For this review, take the finished solid that the model builds, in its own axes (mm). A direction names the side the tool comes from. Round coordinates to 2 decimals unless told otherwise and drop trailing zeros. Order: outer loops, then holes, each group sorted by start corner. A loop starts at its lowest first (then second) coordinate and runs counter-clockwise, first axis right, second up. Notation, with made-up numbers: (53.5, -3.5) - (65.5, -3.5) arc R21 cw to (65.5, 28.5) - close; hole circle Ø8 at (73, 4.5). An arc over 180 degrees is marked (long way). One line per item, written item: value.
Autodesk Inventor part; units mm, degrees
ref_plane "YZ Plane" through (0, 0, 0) normal (1, 0, 0) x (0, 1, 0)
ref_plane "XZ Plane" through (0, 0, 0) normal (0, 1, 0) x (-1, 0, 0)
ref_plane "XY Plane" through (0, 0, 0) normal (0, 0, 1) x (1, 0, 0)
sketch "Sketch1" plane through (0, 0, 0) normal (0, 1, 0) x (-1, 0, 0)
  line L0 (53.975, 34.925) -> (-53.975, 34.925)
  line L1 (-53.975, 34.925) -> (-53.975, -34.925)
  line L2 (-53.975, -34.925) -> (53.975, -34.925)
  line L3 (53.975, -34.925) -> (53.975, 34.925)
  line L4 (0, -48.895) -> (0, 48.895)
  line L5 (-75.565, 0) -> (75.565, 0)
  point P0 (0, 0)
  dimension "d0" = 69.85
  dimension "d1" = 107.95
extrude "Extrusion1" add sketch "Sketch1" along normal blind 50.8
sketch "Sketch2" plane through (0, 50.8, 0) normal (0, 1, 0) x (1, 0, 0)
  line L0 (-53.975, -34.925) -> (53.975, -34.925)
  line L1 (53.975, -34.925) -> (53.975, 34.925)
  line L2 (53.975, 34.925) -> (-53.975, 34.925)
  line L3 (-53.975, 34.925) -> (-53.975, -34.925)
  line L4 (15.875, -9.525) -> (41.275, -9.525)
  line L5 (41.275, -9.525) -> (41.275, 9.525)
  line L6 (41.275, 9.525) -> (15.875, 9.525)
  line L7 (15.875, 9.525) -> (15.875, -9.525)
  line L8 (75.565, 0) -> (-75.565, 0)
  circle A0 centre (28.575, 0) radius 3.175
  line L9 (28.575, -9.525) -> (28.575, 9.525) construction
  point P0 (0, 0)
  dimension "d4" = 25.4
  dimension "d5" = 19.05
  dimension "d7" = 6.35
  dimension "d29" = 12.7
extrude "Extrusion2" add sketch "Sketch2" along normal blind 28.575 contours L8 A0 L5 L4 L7 | L7 L6 L5 L8 A0
sketch "Sketch3" plane through (-53.975, 0, -34.925) normal (-1, 0, 0) x (0, 0, 1)
  line L0 (0, 0) -> (69.85, 0)
  line L1 (69.85, 0) -> (69.85, 50.8)
  line L2 (0, 50.8) -> (69.85, 50.8)
  line L3 (0, 0) -> (0, 50.8)
  line L4 (65.278, 4.572) -> (4.572, 4.572)
  line L5 (4.572, 4.572) -> (4.572, 46.228)
  line L6 (4.572, 46.228) -> (65.278, 46.228)
  line L7 (65.278, 46.228) -> (65.278, 4.572)
  point P0 (34.925, 0)
  dimension "d10" = 4.572
extrude "Extrusion3" cut sketch "Sketch3" against normal up to next contours L4 L5 L6 L7
sketch "Sketch4" plane through (0, 0, 0) normal (0, -1, 0) x (1, 0, 0)
  line L0 (-53.975, 34.925) -> (53.975, 34.925)
  line L1 (-53.975, -34.925) -> (-53.975, 34.925)
  line L2 (53.975, -34.925) -> (-53.975, -34.925)
  line L3 (53.975, 34.925) -> (53.975, -34.925)
  line L4 (9.525, -19.05) -> (47.625, -19.05)
  line L5 (47.625, -19.05) -> (47.625, 19.05)
  line L6 (47.625, 19.05) -> (9.525, 19.05)
  line L7 (9.525, 19.05) -> (9.525, -19.05)
  line L8 (-79.233, 0) -> (97.5728, 0) construction
  arc A0 (-41.275, 9.525) -> (-41.275, -9.525) centre (-41.275, 0) ccw
  arc A1 (-15.875, -9.525) -> (-15.875, 9.525) centre (-15.875, 0) ccw
  arc A2 (-41.275, -23.3807) -> (-41.275, -27.4193) centre (-41.275, -25.4) ccw
  arc A3 (-15.875, -27.4193) -> (-15.875, -23.3807) centre (-15.875, -25.4) ccw
  arc A4 (-41.275, 27.4193) -> (-41.275, 23.3807) centre (-41.275, 25.4) ccw
  arc A5 (-15.875, 23.3807) -> (-15.875, 27.4193) centre (-15.875, 25.4) ccw
  line L9 (-28.575, -34.925) -> (-28.575, 34.925) construction
  line L10 (-41.275, -25.4) -> (-41.275, 25.4) construction
  line L11 (-41.275, -27.4193) -> (-15.875, -27.4193)
  line L12 (-15.875, -23.3807) -> (-41.275, -23.3807)
  line L13 (-41.275, 23.3807) -> (-15.875, 23.3807)
  line L14 (-15.875, 27.4193) -> (-41.275, 27.4193)
  line L15 (-41.275, -9.525) -> (-15.875, -9.525)
  line L16 (-15.875, 9.525) -> (-41.275, 9.525)
  circle A6 centre (28.575, 0) radius 12.7
  line L17 (28.575, 19.05) -> (28.575, -19.05) construction
  point P0 (0, 0)
  dimension "d13" = 38.1
  dimension "d14" = 6.35
  dimension "d15" = 4.0386
  dimension "d16" = 25.4
  dimension "d17" = 25.4
  dimension "d18" = 12.7
  dimension "d19" = 19.05
  dimension "d22" = 25.4
extrude "Extrusion4" cut sketch "Sketch4" against normal up to surface (4.572 mm away) contours L16 A1 L15 A0 | L12 A3 L11 A2 | L14 A5 L13 A4
extrude "Extrusion5" add sketch "Sketch4" along normal blind 215.9 contours L7 L6 L5 L4
sketch "Sketch5" plane through (41.275, 50.8, -9.525) normal (0, 0, -1) x (-1, 0, 0)
  line L0 (25.4, 0) -> (0, 0)
  line L1 (25.4, 0) -> (25.4, 28.575)
  line L2 (0, 28.575) -> (25.4, 28.575)
  line L3 (0, 0) -> (0, 28.575)
  circle A0 centre (12.7, 18.415) radius 3.175
  line L4 (25.4, 28.575) -> (0, 28.575) construction
  line L5 (12.7, 28.575) -> (12.7, 0) construction
  point P0 (41.275, -50.8)
  dimension "d25" = 6.35
  dimension "d26" = 10.16
extrude "Extrusion6" cut sketch "Sketch5" against normal up to surface (19.05 mm away) contours A0
properties part number "DART Actuator"
Item 1: For P1, Ø1.9, axis at x = 27, z = -0.5, coming from the +Y side; P2, Ø6, axis at y = -118.5, z = -11, coming from the -X side (3 decimals); P3, Ø7.5, axis at x = 31, y = 63, coming from the -Z side (3 decimals), all flat-tipped, find the tip position at first contact; note any pin that passes through.
Returned:
P1: y = 50.8
P2: x = 9.525
P3: z = -9.525
Item 2: Take a section at C-C (x = 35). Write out the cut boundary in (y, z) (3 decimals).
Returned:
outline: (-215.9, -19.05) - (0, -19.05) - (0, -34.925) - (50.8, -34.925) - (50.8, -9.525) - (79.375, -9.525) - (79.375, 9.525) - (50.8, 9.525) - (50.8, 34.925) - (0, 34.925) - (0, 19.05) - (-215.9, 19.05) - (-215.9, 10.955) - (0, 10.955) - (0, -10.955) - (-215.9, -10.955) - close; hole (4.572, -30.353) - (46.228, -30.353) - (46.228, 30.353) - (4.572, 30.353) - close
Item 3: Machinability: for faces 5 (the flat face through (28, -106, -19.05)), 6 (the flat face through (-1, 26, 30.353)), 7 (the flat face through (47.625, -106, 0)), 8 (the flat face through (28, 65, 9.525)), 9 (the cylindrical face through (28.162, 59.879, 3.148)), which of the approach directions +Z, -Z, +X, -X, +Y, -Y give a long, thin tool a straight path to every point of the face, cutting with its end or side? Answer none if there is none.
Returned:
face 5: -Z, +X, -X, -Y
face 6: +X, -X
face 7: +Z, -Z, +X, -Y
face 8: +Z, +X, -X, +Y
face 9: +Y
Item 4: Take a section at B-B (y = -137.5). Write out the cut boundary in (x, z) (3 decimals).
Returned:
outline: (9.525, -19.05) - (47.625, -19.05) - (47.625, 19.05) - (9.525, 19.05) - close; hole circle Ø25.4 at (28.575, 0)
Item 5: Wall thickness on line 1 (X direction, y = 72.25, z = 0) (3 decimals); line 2 (Y direction, x = -31, z = -21.5); line 3 (Z direction, x = 46.5, y = 18.5) (3 decimals): over which ranges is each line inside the solid? List them lowest first.
Returned:
line 1: 15.875 to 25.4, 31.75 to 41.275
line 2: 0 to 4.57, 46.23 to 50.8
line 3: -34.925 to -30.353, 30.353 to 34.925
Item 6: Take a section at A-A (y = 14). Write out the cut boundary in (x, z) (3 decimals).
Returned:
outline: (-53.975, -34.925) - (53.975, -34.925) - (53.975, -30.353) - (-53.975, -30.353) - close; (-53.975, 30.353) - (53.975, 30.353) - (53.975, 34.925) - (-53.975, 34.925) - close
Item 7: Take a section at D-D (x = -9). Write out the cut boundary in (y, z) (3 decimals), plus the area to 3 significant figures.
Returned:
outline: (0, -34.925) - (50.8, -34.925) - (50.8, 34.925) - (0, 34.925) - (0, 6.592) - (4.572, 6.592) - (4.572, 30.353) - (46.228, 30.353) - (46.228, -30.353) - (4.572, -30.353) - (4.572, -6.592) - (0, -6.592) - close
area: 959 mm^2
Item 8: The part is to be moulded in two halves that separate along Z. For faces 1 (the flat face through (-1, 4.572, 0)), 2 (the flat face through (41.275, 65, 0)), 3 (the flat face through (29, 50.8, 0)), 4 (the flat face through (1, 25, -34.925)), say which applies: +Z half, -Z half, draft (parallel to the pull), parting line (faces both ways), or undercut.
Returned:
face 1: undercut
face 2: draft
face 3: undercut
face 4: -Z half
